Check sheet for the modelled part. Datum: model origin and axes. Units: mm. Face numbers are marked on the shaded views. A direction names the side the tool comes from. Give positions to 0.01 mm unless a question says otherwise; leave off trailing zeros. Loops run counter-clockwise (first coordinate to the right, second up) from the corner with the lowest first, then second, coordinate; pieces in that order, holes last. Notation, with made-up numbers: M 80.5,-23.75 L 122.5,-23.75 A20 ccw 122.5,7.25 Z; hole C 51.5,51 d8. An arc over 180 degrees is marked long. One line per question, with ' | ' between items. Start each with the question number.
from build123d import *

# Parameters (mm, degrees)
SKETCH1_W      = 528.8
SKETCH1_H      = 50
EXTRUDE2_DEPTH = 10
SKETCH2_R      = 7.5
EXTRUDE3_DEPTH = 50
SKETCH3_W      = 9.599831793
SKETCH3_H      = 14.484799928
EXTRUDE4_DEPTH = 50
SKETCH5_R      = 4.55017582
EXTRUDE5_DEPTH = 50
EXTRUDE6_DEPTH = 10


with BuildPart() as part:
    # Sketch1 → Extrude2 (new body)
    with BuildSketch(Plane(origin=(0, 0, 0), x_dir=(1, 0, 0), z_dir=(0, 1, 0))):
        Rectangle(SKETCH1_W, SKETCH1_H)
    extrude(amount=EXTRUDE2_DEPTH)

    # Sketch2 → Extrude3 (add)
    with BuildSketch(Plane.XY.offset(25)):
        with Locations((264.4, 5)):
            Circle(SKETCH2_R)
    extrude(amount=-EXTRUDE3_DEPTH)

    # Sketch3 → Extrude4 (add)
    with BuildSketch(Plane.XY.offset(25)):
        with Locations((269.199915896, 12.242399964)):
            Rectangle(SKETCH3_W, SKETCH3_H)
    extrude(amount=-EXTRUDE4_DEPTH)

    # Sketch5 → Extrude5 (cut)
    with BuildSketch(Plane.XY.offset(25)):
        with Locations((264.4, 5)):
            Circle(SKETCH5_R)
    extrude(amount=-EXTRUDE5_DEPTH, mode=Mode.SUBTRACT)

    # Sketch6 → Extrude6 (add)
    with BuildSketch(Plane(origin=(0, 0, 0), x_dir=(1, 0, 0), z_dir=(0, 1, 0))):
        with BuildLine():
            Line((-48.968651803, 29.346426348), (-48.968651803, -42.454090949))
            add(Edge.make_bspline(
                [(-48.968651803, -42.454090949), (-48.968651803, -44.874729009), (-46.548013742, -44.874729009)],
                knots=[5.620479698, 5.620479698, 5.620479698, 6.945890916, 6.945890916, 6.945890916], degree=2, weights=[1, 0.788330488, 1]))
            Line((-46.548013742, -44.874729009), (25.252503554, -44.874729009))
            add(Edge.make_bspline(
                [(25.252503554, -44.874729009), (27.673141615, -44.874729009), (27.673141615, -42.454090949)],
                knots=[5.620479698, 5.620479698, 5.620479698, 6.945890916, 6.945890916, 6.945890916], degree=2, weights=[1, 0.788330488, 1]))
            Line((27.673141615, -42.454090949), (27.673141615, 29.346426348))
            add(Edge.make_bspline(
                [(27.673141615, 29.346426348), (27.673141615, 31.767064408), (25.252503554, 31.767064408)],
                knots=[5.620479698, 5.620479698, 5.620479698, 6.945890916, 6.945890916, 6.945890916], degree=2, weights=[1, 0.788330488, 1]))
            Line((25.252503554, 31.767064408), (-46.548013742, 31.767064408))
            add(Edge.make_bspline(
                [(-46.548013742, 31.767064408), (-48.968651803, 31.767064408), (-48.968651803, 29.346426348)],
                knots=[5.620479698, 5.620479698, 5.620479698, 6.945890916, 6.945890916, 6.945890916], degree=2, weights=[1, 0.788330488, 1]))
        make_face()
    extrude(amount=EXTRUDE6_DEPTH)


solid = part.part
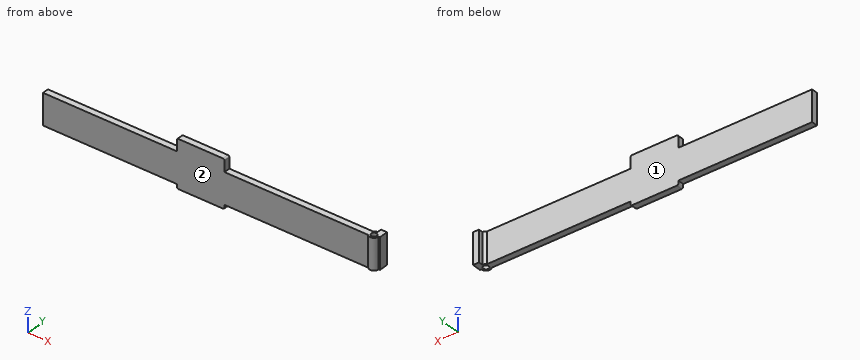
Q1. Depth check by flat-ended pin: P1, Ø5, axis at x = -106.5, y = 6.5, coming from the -Z side; P2, Ø5, axis at x = 147.5, y = 11.5, coming from the +Z side; P3, Ø5, axis at y = 3.5, z = 37, coming from the +X side. Enter the tip coordinate at first touch or a pass-through.
Q2. Access from +Z, -Z, +X, -X, +Y, -Y to the whole of each face (thin tool, end or side, straight path). Record for the marked faces 1 and 2.
Q3. Cross-section at B-B (x = -105). Record the cut outline in (y, z), and give its area (3 significant figures).
Q4. Material ranges on probe 1 along Y at (x, z) = (264, -12); probe 2 along X at (y, z) = (4.5, 1.5); probe 3 along Y at (x, z) = (-5, 38.5), recorded low to high. Write a range as from..to.
Q5. Cross-section at A-A (z = 15). Record the cut outline in (x, y).
Q6. Cross-section at C-C (x = -1). Record the cut outline in (y, z), and give its area (3 significant figures).
Solved:
1) P1: stops at z = -25 | P2: stops at z = 25 | P3: stops at x = 27.67
2) face 1: +Z, -Z, -X, +Y | face 2: +Z, -Z, -X, -Y
3) outline: M 0,-25 L 10,-25 L 10,25 L 0,25 Z | area: 500 mm²
4) probe 1: y = -2.49..0.47, 9.53..12.49 | probe 2: x = -264.4..259.88, 268.92..271.88 | probe 3: y = 0..10
5) outline: M -264.4,0 L 258.81,0 A7.5 ccw 271.9,5 L 274,5 L 274,19.48 L 264.4,19.48 L 264.4,12.5 A7.5 ccw 258.81,10 L -264.4,10 Z; hole C 264.4,5 d9.1
6) outline: M 0,-31.77 L 10,-31.77 L 10,44.87 L 0,44.87 Z | area: 766 mm²
